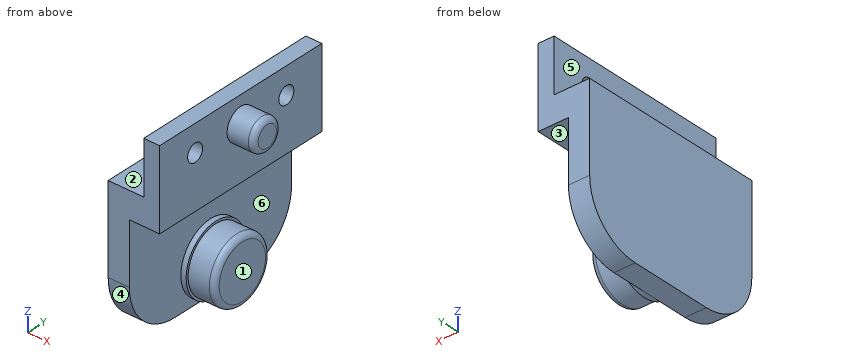
```python
from build123d import *

# Parameters (mm, degrees)
SKETCH4_W                = 12.46
SKETCH4_H                = 17.25
BOSS_EXTRUDE3_DEPTH      = 6
SKETCH8_R                = 12.546781182
SKETCH8_R_2              = 11.15
BOSS_EXTRUDE6_DEPTH      = 8.3
BOSS_EXTRUDE6_DEPTH_BACK = 17.25
BOSS_EXTRUDE4_DEPTH      = 17.25
SKETCH6_R                = 0.75
CUT_EXTRUDE1_DEPTH       = 5
CHAMFER1_SIZE            = 0.5
CHAMFER1_SIZE2           = 0.866025404
SKETCH10_W               = 12.46
SKETCH10_H               = 23.7
CUT_EXTRUDE3_DEPTH       = 17.25
BOSS_EXTRUDE7_DEPTH      = 8.3
BOSS_EXTRUDE9_DEPTH      = 10
SKETCH20_R               = 11.15
SKETCH20_R_2             = 7.15
BOSS_EXTRUDE11_DEPTH     = 8.3
SKETCH21_R               = 10.15
SKETCH21_R_2             = 7.15
CUT_EXTRUDE7_DEPTH       = 1.3
SKETCH11_W               = 10
SKETCH11_H               = 2
CUT_EXTRUDE4_DEPTH       = 23.7
CUT_EXTRUDE8_REACH       = 37.55
SKETCH25_W               = 12.46
SKETCH25_H               = 6
BOSS_EXTRUDE10_DEPTH     = 35.55
SKETCH18_W               = 21.5
SKETCH18_H               = 11.438292938
CUT_EXTRUDE5_DEPTH       = 2
SKETCH19_R               = 3.5
CUT_EXTRUDE6_DEPTH       = 43.5
CUT_EXTRUDE6_DEPTH_BACK  = 3
FILLET1_R                = 10
SKETCH22_R               = 6.5
BOSS_EXTRUDE12_DEPTH     = 5
SKETCH23_R               = 6.075
BOSS_EXTRUDE13_DEPTH     = 5
FILLET2_R                = 1
BOSS_EXTRUDE14_DEPTH     = 2
CUT_EXTRUDE9_REACH       = 46.5
SKETCH27_R               = 0.75
CUT_EXTRUDE10_DEPTH      = 36.55
SKETCH29_W               = 3
SKETCH29_H               = 35.55
BOSS_EXTRUDE15_DEPTH     = 10
SKETCH30_R               = 3
BOSS_EXTRUDE16_DEPTH     = 5
FILLET3_R                = 1
SKETCH31_R               = 1.65
CUT_EXTRUDE11_DEPTH      = 23.25


with BuildPart() as part:
    # Sketch4 → Boss-Extrude3 (new body)
    with BuildSketch(Plane.XY):
        with Locations((0, -1.35)):
            Rectangle(SKETCH4_W, SKETCH4_H)
    extrude(amount=BOSS_EXTRUDE3_DEPTH)



with BuildPart() as body_2:
    # Sketch8 → Boss-Extrude6 (new body, two sides)
    with BuildSketch(Plane(origin=(0, -9.975, 0), x_dir=(-1, 0, 0), z_dir=(0, -1, 0))) as boss_extrude6_sk:
        with Locations((0, -23.55)):
            Circle(SKETCH8_R)
        with Locations((0, -23.55)):
            Circle(SKETCH8_R_2, mode=Mode.SUBTRACT)
    extrude(amount=BOSS_EXTRUDE6_DEPTH)
    extrude(boss_extrude6_sk.sketch, amount=-BOSS_EXTRUDE6_DEPTH_BACK)


with BuildPart() as part_1:
    add(part.part)

    add(body_2.part)  # Boss-Extrude4 merges body 2
    # Sketch5 → Boss-Extrude4 (add)
    with BuildSketch(Plane(origin=(0, 7.275, 0), x_dir=(1, 0, 0), z_dir=(0, 1, 0))):
        with BuildLine():
            Line((12.546781182, -23.55), (12.546781182, 0))
            Line((12.546781182, 0), (6.23, 0))
            Line((6.23, 0), (6.23, -29.7))
            Line((6.23, -29.7), (-6.23, -29.7))
            Line((-6.23, -29.7), (-6.23, 0))
            Line((-6.23, 0), (-12.546781182, 0))
            Line((-12.546781182, 0), (-12.546781182, -23.55))
            ThreePointArc((-12.546781182, -23.55), (0, -36.096781182), (12.546781182, -23.55))
        make_face()
    extrude(amount=-BOSS_EXTRUDE4_DEPTH)

    # Sketch6 → Cut-Extrude1 (cut)
    with BuildSketch(Plane(origin=(0, 7.275, 0), x_dir=(1, 0, 0), z_dir=(0, 1, 0))):
        with Locations((0, -3.6)):
            Circle(SKETCH6_R)
        with Locations((0, -32.1)):
            Circle(SKETCH6_R)
    extrude(amount=-CUT_EXTRUDE1_DEPTH, mode=Mode.SUBTRACT)

    # Chamfer1
    chamfer1_edges = [part_1.edges().sort_by_distance(p)[0] for p in [
        (-0.75, 7.275, 3.6),
        (-0.75, 7.275, 32.1),
    ]]
    chamfer1_side = [part_1.faces().sort_by_distance(p)[0] for p in [
        (0, 7.275, 35.657160381),
    ]]
    chamfer(chamfer1_edges, length=CHAMFER1_SIZE, length2=CHAMFER1_SIZE2, reference=chamfer1_side[0])

    # Sketch10 → Cut-Extrude3 (cut)
    with BuildSketch(Plane(origin=(0, 7.275, 0), x_dir=(1, 0, 0), z_dir=(0, 1, 0))):
        with Locations((0, -17.85)):
            Rectangle(SKETCH10_W, SKETCH10_H)
    extrude(amount=-CUT_EXTRUDE3_DEPTH, mode=Mode.SUBTRACT)

    # Sketch13 → Boss-Extrude7 (add)
    with BuildSketch(Plane.XZ.offset(18.275)):
        with BuildLine():
            Line((-12.546781182, 23.55), (-12.546781182, 0))
            Line((-12.546781182, 0), (12.546781182, 0))
            Line((12.546781182, 0), (12.546781182, 23.55))
            ThreePointArc((12.546781182, 23.55), (0, 11.003218818), (-12.546781182, 23.55))
        make_face()
    extrude(amount=-BOSS_EXTRUDE7_DEPTH)

    # Sketch15 → Boss-Extrude9 (add)
    with BuildSketch(Plane(origin=(0, 7.275, 0), x_dir=(1, 0, 0), z_dir=(0, 1, 0))):
        with BuildLine():
            Line((-12.546781182, 0), (12.546781182, 0))
            Line((12.546781182, 0), (12.546781182, -23.55))
            ThreePointArc((12.546781182, -23.55), (0, -36.096781182), (-12.546781182, -23.55))
            Line((-12.546781182, -23.55), (-12.546781182, 0))
        make_face()
        with BuildLine():
            Line((-6.23, -0.8), (6.23, -0.8))
            Line((6.23, -0.8), (6.23, -33))
            ThreePointArc((6.23, -33), (5.790660172, -34.060660172), (4.73, -34.5))
            Line((4.73, -34.5), (-4.73, -34.5))
            ThreePointArc((-4.73, -34.5), (-5.790660172, -34.060660172), (-6.23, -33))
            Line((-6.23, -33), (-6.23, -0.8))
        make_face(mode=Mode.SUBTRACT)
    extrude(amount=BOSS_EXTRUDE9_DEPTH)

    # Sketch20 → Boss-Extrude11 (add)
    with BuildSketch(Plane.XZ.offset(18.275)):
        with Locations((0, 23.55)):
            Circle(SKETCH20_R)
        with Locations((0, 23.55)):
            Circle(SKETCH20_R_2, mode=Mode.SUBTRACT)
    extrude(amount=-BOSS_EXTRUDE11_DEPTH)

    # Sketch21 → Cut-Extrude7 (cut)
    with BuildSketch(Plane.XZ.offset(18.275)):
        with Locations((0, 23.55)):
            Circle(SKETCH21_R)
        with Locations((0, 23.55)):
            Circle(SKETCH21_R_2, mode=Mode.SUBTRACT)
    extrude(amount=-CUT_EXTRUDE7_DEPTH, mode=Mode.SUBTRACT)

    # Sketch11 → Cut-Extrude4 (cut)
    with BuildSketch(Plane.XY.offset(29.7)):
        with Locations((0, -10.975)):
            Rectangle(SKETCH11_W, SKETCH11_H)
    extrude(amount=-CUT_EXTRUDE4_DEPTH, mode=Mode.SUBTRACT)

    # Sketch25 → Cut-Extrude8 (cut, up to next)
    with BuildSketch(Plane.XZ.offset(18.275), mode=Mode.PRIVATE) as cut_extrude8_sk1:
        with Locations((0, 9)):
            Rectangle(SKETCH25_W, SKETCH25_H)
    cut_extrude8_tool1 = extrude(cut_extrude8_sk1.sketch, amount=-CUT_EXTRUDE8_REACH, mode=Mode.PRIVATE) & part_1.part
    add(cut_extrude8_tool1.solids().sort_by_distance((0, -18.275, 9))[0], mode=Mode.SUBTRACT)

    # Sketch17 → Boss-Extrude10 (add)
    with BuildSketch(Plane(origin=(0, 17.275, 0), x_dir=(1, 0, 0), z_dir=(0, 1, 0))):
        Polygon((22.25, 26.5), (22.25, 0), (-22.25, 0), (-22.25, 26.5), (-18.25, 26.5), (-18.25, 5), (18.25, 5), (18.25, 26.5), align=None)
    extrude(amount=-BOSS_EXTRUDE10_DEPTH)

    # Sketch18 → Cut-Extrude5 (cut)
    with BuildSketch(Plane.ZY.offset(-18.25)):
        with Locations((-15.75, -0.5)):
            Rectangle(SKETCH18_W, SKETCH18_H)
    extrude(amount=-CUT_EXTRUDE5_DEPTH, mode=Mode.SUBTRACT)

    # Sketch19 → Cut-Extrude6 (cut, two sides)
    with BuildSketch(Plane.ZY.offset(-20.25)) as cut_extrude6_sk:
        with Locations((-20, -0.5)):
            Circle(SKETCH19_R)
    extrude(amount=CUT_EXTRUDE6_DEPTH, mode=Mode.SUBTRACT)
    extrude(cut_extrude6_sk.sketch, amount=-CUT_EXTRUDE6_DEPTH_BACK, mode=Mode.SUBTRACT)

    # Fillet1
    fillet1_edges = [part_1.edges().sort_by_distance(p)[0] for p in [
        (20.25, 17.275, -26.5),
        (-20.25, 17.275, -26.5),
        (-20.25, -18.275, -26.5),
        (20.25, -18.275, -26.5),
    ]]
    fillet(fillet1_edges, radius=FILLET1_R)

    # Sketch22 → Boss-Extrude12 (add)
    with BuildSketch(Plane.ZY.offset(22.25)):
        with Locations((-20, -0.5)):
            Circle(SKETCH22_R)
    extrude(amount=-BOSS_EXTRUDE12_DEPTH)

    # Sketch23 → Boss-Extrude13 (add)
    with BuildSketch(Plane(origin=(-17.25, 0, 0), x_dir=(0, 0, -1), z_dir=(1, 0, 0))):
        with Locations((20, -0.5)):
            Circle(SKETCH23_R)
    extrude(amount=BOSS_EXTRUDE13_DEPTH)

    # Fillet2
    fillet2_edges = [part_1.edges().sort_by_distance(p)[0] for p in [
        (-12.25, -0.5, -13.925),
    ]]
    fillet(fillet2_edges, radius=FILLET2_R)

    # Sketch26 → Boss-Extrude14 (add)
    with BuildSketch(Plane.ZY.offset(-20.25)):
        Polygon((-5, 2), (-20, 2.6585), (-26.5, 2.94385), (-26.5, 5.219146469), (-5, 5.219146469), align=None)
        Polygon((-20, -3.6585), (-5, -3), (-5, -6.219146469), (-26.5, -6.219146469), (-26.5, -3.94385), align=None)
    extrude(amount=BOSS_EXTRUDE14_DEPTH)

    # Sketch27 → Cut-Extrude9 (cut, up to next)
    with BuildSketch(Plane(origin=(22.25, 0, 0), x_dir=(0, 0, -1), z_dir=(1, 0, 0)), mode=Mode.PRIVATE) as cut_extrude9_sk1:
        with Locations((10, -0.5)):
            Circle(SKETCH27_R)
    cut_extrude9_tool1 = extrude(cut_extrude9_sk1.sketch, amount=-CUT_EXTRUDE9_REACH, mode=Mode.PRIVATE) & part_1.part
    add(cut_extrude9_tool1.solids().sort_by_distance((22.25, -0.5, -10))[0], mode=Mode.SUBTRACT)

    # Sketch28 → Cut-Extrude10 (cut, through all)
    with BuildSketch(Plane(origin=(0, 17.275, 0), x_dir=(1, 0, 0), z_dir=(0, 1, 0))):
        Polygon((-12.546781182, 11.805014222), (-12.546781182, -42.756283402), (39.689088419, -42.756283402), (38.70358058, 30.977621269), (-8.600795685, 28.379464239), align=None)
    extrude(amount=-CUT_EXTRUDE10_DEPTH, mode=Mode.SUBTRACT)

    # Sketch29 → Boss-Extrude15 (add)
    with BuildSketch(Plane.XY):
        with Locations((-14.046781182, -0.5)):
            Rectangle(SKETCH29_W, SKETCH29_H)
    extrude(amount=BOSS_EXTRUDE15_DEPTH)

    # Sketch30 → Boss-Extrude16 (add)
    with BuildSketch(Plane(origin=(-12.546781182, 0, 0), x_dir=(0, 0, -1), z_dir=(1, 0, 0))):
        with Locations((-5, -0.5)):
            Circle(SKETCH30_R)
    extrude(amount=BOSS_EXTRUDE16_DEPTH)

    # Fillet3
    fillet3_edges = [part_1.edges().sort_by_distance(p)[0] for p in [
        (-7.546781182, -0.5, 8),
    ]]
    fillet(fillet3_edges, radius=FILLET3_R)

    # Sketch31 → Cut-Extrude11 (cut, through all)
    with BuildSketch(Plane(origin=(0, 0, 0), x_dir=(0, 0, -1), z_dir=(1, 0, 0))):
        with Locations((-5, 9.5)):
            Circle(SKETCH31_R)
        with Locations((-5, -10.5)):
            Circle(SKETCH31_R)
    extrude(amount=-CUT_EXTRUDE11_DEPTH, mode=Mode.SUBTRACT)


solid = part_1.part
```
Check sheet for the modelled part. Datum: model origin and axes. Units: mm. Face numbers are marked on the shaded views. A direction names the side the tool comes from. Round coordinates to 2 decimals unless told otherwise and drop trailing zeros. Loops run counter-clockwise (first coordinate to the right, second up) from the corner with the lowest first, then second, coordinate; pieces in that order, holes last. Notation, with made-up numbers: (-15.75, 85.5) -> (8.25, 85.5) arc R4 ccw to (8.25, 92.5) -> close; hole circle Ø11 at (61, 47.25). An arc over 180 degrees is marked (long way). Write item = value, one per line. Start each with the question number.
1) Sectioned sample at A-A, the plane z = 5. Record the cut outline in (x, y) (3 decimals), plus the area to 3 significant figures.
2) Set-up check for the marked faces 1, 2 and 3: record each of +Z, -Z, +X, -X, +Y, -Y from which the full face is reachable in a straight line by a thin tool's end or side.
3) Release check for a two-part mould opening along Z. For the marked faces 4, 5 and 6 record: released by +Z, released by -Z, zero draft, split by the parting line, or undercut.
4) Gauge pin test, flat ends, axial feed: pin 1 Ø3.5 at (x, y) = (-19, 2) entering from +Z; pin 2 Ø11 at (y, z) = (-7.5, -15) entering from +X; pin 3 Ø4 at (x, z) = (-13.5, -8) entering from -Y; pin 4 Ø6.5 at (x, y) = (-14, 7.5) entering from -Z. Record the tip position at first contact, or that the pin passes through.
5) Sectioned sample at B-B, the plane y = -10.5. Record the cut outline in (x, z), plus the area to 3 significant figures.
6) Sectioned sample at D-D, the plane x = -9.75. Record the cut outline in (y, z).
7) Thickness scan on probe 1 along Y at (x, z) = (-14, 5) (3 decimals); probe 2 along X at (y, z) = (-14.5, -14); probe 3 along Z at (x, y) = (-21, -0.5). Record the ranges inside material, lowest first.
Results are:
q1.outline = (-15.547, -18.275) -> (-12.547, -18.275) -> (-12.547, -12.15) -> (-15.547, -12.15) -> close; (-15.547, -8.85) -> (-12.547, -8.85) -> (-12.547, -3.5) -> (-8.547, -3.5) arc R1 ccw to (-7.547, -2.5) -> (-7.547, 1.5) arc R1 ccw to (-8.547, 2.5) -> (-12.547, 2.5) -> (-12.547, 7.85) -> (-15.547, 7.85) -> close; (-15.547, 11.15) -> (-12.547, 11.15) -> (-12.547, 17.275) -> (-15.547, 17.275) -> close
q1.area = 116 mm^2
q2.face_1 = -Z, +X, +Y, -Y
q2.face_2 = +Z, -X, +Y, -Y
q2.face_3 = +X, +Y, -Y
q3.face_4 = released by -Z
q3.face_5 = zero draft
q3.face_6 = undercut
q4.pin_1 = 0
q4.pin_2 = -12.25
q4.pin_3 = through
q4.pin_4 = -23.79
q5.outline = (-22.25, -26.25) -> (-18.25, -26.25) -> (-18.25, -5) -> (-12.55, -5) -> (-12.55, 3.35) -> (-15.55, 3.35) -> (-15.55, 0) -> (-22.25, 0) -> close; (-15.55, 6.65) -> (-12.55, 6.65) -> (-12.55, 10) -> (-15.55, 10) -> close
q5.area = 154 mm^2
q6.outline = circle Ø6 at (-0.5, 5)
q7.probe_1 = -18.275 to -12.15, -8.85 to 7.85, 11.15 to 17.275
q7.probe_2 = -22.25 to -18.25
q7.probe_3 = -26.5 to 0
